The model under review builds one solid part; all positions refer to its coordinate system, in mm. Face numbers are marked on the shaded views. A direction names the side the tool comes from. Round coordinates to 2 decimals unless told otherwise and drop trailing zeros. Write each loop counter-clockwise with the first axis right and the second up, starting at its lowest first coordinate (ties: lowest second). Pieces come first, ordered by that corner, then holes. Notation, with made-up numbers: (27.25, 16.25) - (81.25, 16.25) arc R21 cw to (81.25, 33.25) - close; hole circle Ø7 at (54, -26.5). An arc over 180 degrees is marked (long way). Return JSON: item names as keys, results as strings.
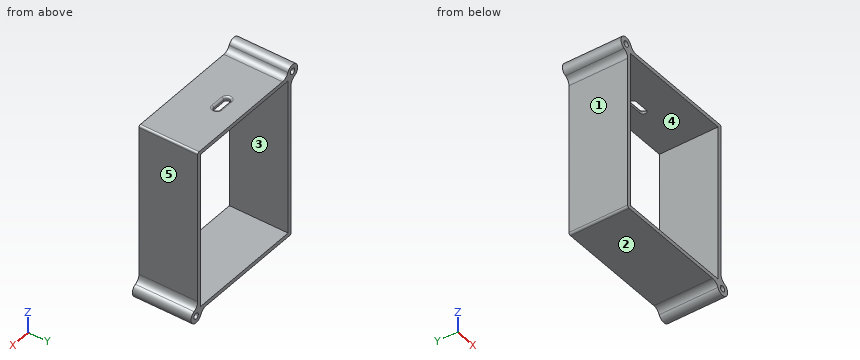
from build123d import *

# Parameters (mm, degrees)
SKETCH1_W           = 64
SKETCH1_H           = 84
SKETCH1_W_2         = 60
SKETCH1_H_2         = 80
BOSS_EXTRUDE1_DEPTH = 30
SKETCH2_R           = 3.5
SKETCH2_R_2         = 1.5
BOSS_EXTRUDE2_DEPTH = 30
CUT_EXTRUDE1_DEPTH  = 30
FILLET2_R           = 1
FILLET3_R           = 4
FILLET4_R           = 1


with BuildPart() as part:
    # Sketch1 → Boss-Extrude1 (new body)
    with BuildSketch(Plane(origin=(0, 0, 0), x_dir=(1, 0, 0), z_dir=(0, 1, 0))):
        with Locations((30, -40)):
            Rectangle(SKETCH1_W, SKETCH1_H)
        with Locations((30, -40)):
            Rectangle(SKETCH1_W_2, SKETCH1_H_2, mode=Mode.SUBTRACT)
    extrude(amount=BOSS_EXTRUDE1_DEPTH)

    # Sketch2 → Boss-Extrude2 (add)
    # profile 1 of 2: a face of its own
    with BuildSketch(Plane(origin=(0, 0, 0), x_dir=(1, 0, 0), z_dir=(0, 1, 0))):
        with Locations((-3.060660172, -83.060660172)):
            Circle(SKETCH2_R)
        with Locations(Location((-3.060660172, -83.060660172, 0), (0, 0, 270))):
            Circle(SKETCH2_R_2, mode=Mode.SUBTRACT)
    # profile 2 of 2: a face of its own
    with BuildSketch(Plane(origin=(0, 0, 0), x_dir=(1, 0, 0), z_dir=(0, 1, 0))):
        with Locations((63.060660172, 3.060660172)):
            Circle(SKETCH2_R)
        with Locations(Location((63.060660172, 3.060660172, 0), (0, 0, 270))):
            Circle(SKETCH2_R_2, mode=Mode.SUBTRACT)
    extrude(amount=BOSS_EXTRUDE2_DEPTH)

    # Sketch4 → Cut-Extrude1 (cut)
    with BuildSketch(Plane.XY.offset(82)):
        with BuildLine():
            Line((30.141314867, 20.2), (26.741314867, 20.2))
            ThreePointArc((26.741314867, 20.2), (25.141314867, 18.6), (26.741314867, 17))
            Line((26.741314867, 17), (30.141314867, 17))
            Line((30.141314867, 17), (33.541314867, 17))
            ThreePointArc((33.541314867, 17), (35.141314867, 18.6), (33.541314867, 20.2))
            Line((33.541314867, 20.2), (30.141314867, 20.2))
        make_face()
    extrude(amount=-CUT_EXTRUDE1_DEPTH, mode=Mode.SUBTRACT)

    # Fillet2
    fillet2_edges = [part.edges().sort_by_distance(p)[0] for p in [
        (30.141314867, 17, 82),
        (35.141314867, 18.6, 82),
        (30.141314867, 20.2, 82),
        (25.141314867, 18.6, 82),
    ]]
    fillet(fillet2_edges, radius=FILLET2_R)

    # Fillet3
    fillet3_edges = [part.edges().sort_by_distance(p)[0] for p in [
        (-2, 15, 79.725244156),
        (59.725244156, 15, -2),
        (0.274755844, 15, 82),
        (62, 15, 0.274755844),
    ]]
    fillet(fillet3_edges, radius=FILLET3_R)

    # Fillet4
    fillet4_edges = [part.edges().sort_by_distance(p)[0] for p in [
        (-2, 15, -2),
        (62, 15, 82),
    ]]
    fillet(fillet4_edges, radius=FILLET4_R)


solid = part.part
(1) Mouldability with a two-part tool opening along X and no side actions: class the marked faces 1, 2 and 3 as released by +X, released by -X, zero draft, split by the parting line, or undercut.
Filled in:
{"face 1": "released by -X", "face 2": "zero draft", "face 3": "undercut"}
(2) Wall thickness on line 1 (Z direction, x = 49, y = 5); line 2 (X direction, y = 25.75, z = 61.5); line 3 (Z direction, x = 2, y = 14.25): over which ranges is each line inside the solid? List them lowest first.
Filled in:
{"line 1": "z = -2 to 0, 80 to 82", "line 2": "x = -2 to 0, 60 to 62", "line 3": "z = -2 to 0, 80 to 82.45"}
(3) Add section C-C (y = 18.6). Write out the cut boundary in (x, z), plus the area to 3 significant figures.
Filled in:
{"outline": "(-4.43, 79.84) arc R4 cw to (-2, 76.16) - (-2, -1) arc R1 ccw to (-1, -2) - (56.16, -2) arc R4 cw to (59.84, -4.43) arc R3.5 ccw (long way) to (64.43, 0.16) arc R4 cw to (62, 3.84) - (62, 81) arc R1 ccw to (61, 82) - (36.14, 82) arc R1 ccw to (35.14, 81) - (35.14, 80) - (60, 80) - (60, 0) - (0, 0) - (0, 80) - (25.14, 80) - (25.14, 81) arc R1 ccw to (24.14, 82) - (3.84, 82) arc R4 cw to (0.16, 84.43) arc R3.5 ccw (long way) to start; hole circle Ø3 at (-3.06, 83.06); hole circle Ø3 at (63.06, -3.06)", "area": "619 mm2"}
(4) Add section A-A (z = 35.5). Write out the cut boundary in (x, y).
Filled in:
{"outline": "(-2, 0) - (0, 0) - (0, 30) - (-2, 30) - close; (60, 0) - (62, 0) - (62, 30) - (60, 30) - close"}
(5) Add section B-B (x = 18.5). Write out the cut boundary in (y, z), plus the area to 3 significant figures.
Filled in:
{"outline": "(0, -2) - (30, -2) - (30, 0) - (0, 0) - close; (0, 80) - (30, 80) - (30, 82) - (0, 82) - close", "area": "120 mm2"}
(6) Add section D-D (y = 13.5). Write out the cut boundary in (x, z).
Filled in:
{"outline": "(-4.43, 79.84) arc R4 cw to (-2, 76.16) - (-2, -1) arc R1 ccw to (-1, -2) - (56.16, -2) arc R4 cw to (59.84, -4.43) arc R3.5 ccw (long way) to (64.43, 0.16) arc R4 cw to (62, 3.84) - (62, 81) arc R1 ccw to (61, 82) - (3.84, 82) arc R4 cw to (0.16, 84.43) arc R3.5 ccw (long way) to start; hole circle Ø3 at (-3.06, 83.06); hole (0, 0) - (60, 0) - (60, 80) - (0, 80) - close; hole circle Ø3 at (63.06, -3.06)"}
(7) Clearance check with flat-ended pins moving along their axes: pin 1 Ø15 at (x, y) = (38, 11) entering from +Z; pin 2 Ø12 at (y, z) = (20, 36) entering from +X; pin 3 Ø9 at (y, z) = (12, 24.5) entering from -X; pin 4 Ø1.8 at (x, z) = (63.06, -3.06) entering from -Y. State where each tip first meets the part, or that it passes through.
Filled in:
{"pin 1": "stops at z = 82", "pin 2": "stops at x = 62", "pin 3": "stops at x = -2", "pin 4": "passes through"}
(8) For the marked faces 4 and 5, list the 3-axis set-ups (+Z, -Z, +X, -X, +Y, -Y) from which the entire face can be reached by the end or side of a thin tool; tool diameter is ignored.
Filled in:
{"face 4": "+Y, -Y", "face 5": "+Z, +X, +Y, -Y"}
